Build history of the part. All positions in model axes, mm. A direction names the side the tool comes from. Round coordinates to 2 decimals unless told otherwise and drop trailing zeros. Loops run counter-clockwise (first coordinate to the right, second up) from the corner with the lowest first, then second, coordinate; pieces in that order, holes last. Notation, with made-up numbers: (40.25, 1) - (54.25, 1) arc R33 ccw to (54.25, 36) - close; hole circle Ø10 at (70.5, 81.5). An arc over 180 degrees is marked (long way). Use a Markdown table: item, result.
from build123d import *

# Parameters (mm, degrees)
SKETCH1_R           = 3
SKETCH1_R_2         = 1
BOSS_EXTRUDE1_DEPTH = 25
SKETCH1_3_R         = 3
BOSS_EXTRUDE2_DEPTH = 2
SKETCH1_4_R         = 1
BOSS_EXTRUDE3_DEPTH = 8.5
BOSS_EXTRUDE4_DEPTH = 2.75


with BuildPart() as part:
    # Sketch1 → Boss-Extrude1 (new body)
    # profile 1 of 3: a face of its own
    with BuildSketch(Plane(origin=(0, 0, 0), x_dir=(1, 0, 0), z_dir=(0, 1, 0))):
        with BuildLine():
            ThreePointArc((-6.614378278, 7.5), (-10, 0), (-6.614378278, -7.5))
            Line((-6.614378278, -7.5), (6.614378278, -7.5))
            ThreePointArc((6.614378278, -7.5), (9.114378278, -4.114378278), (10, 0))
            ThreePointArc((10, 0), (9.114378278, 4.114378278), (6.614378278, 7.5))
            Line((6.614378278, 7.5), (-6.614378278, 7.5))
        make_face()
        Circle(SKETCH1_R, mode=Mode.SUBTRACT)
    # profile 2 of 3: a face of its own
    with BuildSketch(Plane(origin=(0, 0, 0), x_dir=(1, 0, 0), z_dir=(0, 1, 0))):
        Circle(SKETCH1_R)
        Circle(SKETCH1_R_2, mode=Mode.SUBTRACT)
    # profile 3 of 3: a face of its own
    with BuildSketch(Plane(origin=(0, 0, 0), x_dir=(1, 0, 0), z_dir=(0, 1, 0))):
        Circle(SKETCH1_R_2)
    extrude(amount=-BOSS_EXTRUDE1_DEPTH)

    # Sketch1_3 → Boss-Extrude2 (add)
    with BuildSketch(Plane(origin=(0, 0, 0), x_dir=(1, 0, 0), z_dir=(0, 1, 0))):
        with Locations(Location((0, 0, 0), (0, 0, 270))):
            Circle(SKETCH1_3_R)
    extrude(amount=BOSS_EXTRUDE2_DEPTH)

    # Sketch1_4 → Boss-Extrude3 (add)
    with BuildSketch(Plane(origin=(0, 0, 0), x_dir=(1, 0, 0), z_dir=(0, 1, 0))):
        with Locations(Location((0, 0, 0), (0, 0, 270))):
            Circle(SKETCH1_4_R)
    extrude(amount=BOSS_EXTRUDE3_DEPTH)

    # Sketch2 → Boss-Extrude4 (add)
    with BuildSketch(Plane.XZ.offset(25)):
        with BuildLine():
            ThreePointArc((0, 4.95), (-4.719639817, 1.492481156), (-2.846049894, -4.05))
            Line((-2.846049894, -4.05), (0, -4.05))
            Line((0, -4.05), (0, 4.95))
        make_face()
        with BuildLine():
            Line((0, 4.95), (0, -4.05))
            Line((0, -4.05), (2.846049894, -4.05))
            ThreePointArc((2.846049894, -4.05), (4.392632865, -2.281945773), (4.95, 0))
            ThreePointArc((4.95, 0), (3.500178567, 3.500178567), (0, 4.95))
        make_face()
    extrude(amount=BOSS_EXTRUDE4_DEPTH)


solid = part.part
Q1. Drop flat-ended pins along their axis: pin 1 (5 mm diameter, centred on x = -0.5, z = -1, fed in from +Y); pin 2 (2 mm diameter, centred on x = 0.5, y = -27, fed in from -Z); pin 3 (5 mm diameter, centred on x = -6, z = 2, fed in from +Y); pin 4 (1 mm diameter, centred on y = -19, z = -1, fed in from -X). Give the stop position or say it passes through.
Results found:
| item | result |
|---|---|
| pin 1 | stops at y = 8.5 |
| pin 2 | stops at z = -4.05 |
| pin 3 | stops at y = 0 |
| pin 4 | stops at x = -9.99 |
Q2. Probe line 1 (Y direction, x = -0.75, z = -5.25); line 2 (X direction, y = 2.5, z = 0); line 3 (Y direction, x = -1, z = -2.25). List the from-to ranges inside material, lowest first.
Results found:
| item | result |
|---|---|
| line 1 | y = -25 to 0 |
| line 2 | x = -1 to 1 |
| line 3 | y = -27.75 to 2 |
Q3. Cut at B-B, the plane z = -6. List the corners of the cut face in (x, y), plus the area to 3 significant figures.
Results found:
| item | result |
|---|---|
| outline | (-8, -25) - (8, -25) - (8, 0) - (-8, 0) - close |
| area | 400 mm2 |
Q4. Cut at D-D, the plane z = -1.5. List the corners of the cut face in (x, y), plus the area to 3 significant figures.
Results found:
| item | result |
|---|---|
| outline | (-9.89, -25) - (-4.72, -25) - (-4.72, -27.75) - (4.72, -27.75) - (4.72, -25) - (9.89, -25) - (9.89, 0) - (2.6, 0) - (2.6, 2) - (-2.6, 2) - (-2.6, 0) - (-9.89, 0) - close |
| area | 531 mm2 |
Q5. Cut at C-C, the plane x = -8. List the corners of the cut face in (y, z).
Results found:
| item | result |
|---|---|
| outline | (-25, -6) - (0, -6) - (0, 6) - (-25, 6) - close |
Q6. Which spindle directions (+Z, -Z, +X, -X, +Y, -Y) get a long thin tool onto all of the face, cutting with end or side? Do faces 1 (the face through (0, -25, -5)), 2 (the face through (1, 2, -1)), 3 (the face through (0, -27.75, 1)), 4 (the face through (0, -26, -4.05)), 5 (the face through (0, 8.5, 0)). Say none if no direction does.
Results found:
| item | result |
|---|---|
| face 1 | -Y |
| face 2 | +Y |
| face 3 | +Z, -Z, +X, -X, -Y |
| face 4 | -Z, +X, -X, -Y |
| face 5 | +Z, -Z, +X, -X, +Y |
Q7. Cut at A-A, the plane y = -10. List the corners of the cut face in (x, z).
Results found:
| item | result |
|---|---|
| outline | (-6.61, -7.5) - (6.61, -7.5) arc R10 ccw to (6.61, 7.5) - (-6.61, 7.5) arc R10 ccw to start |
